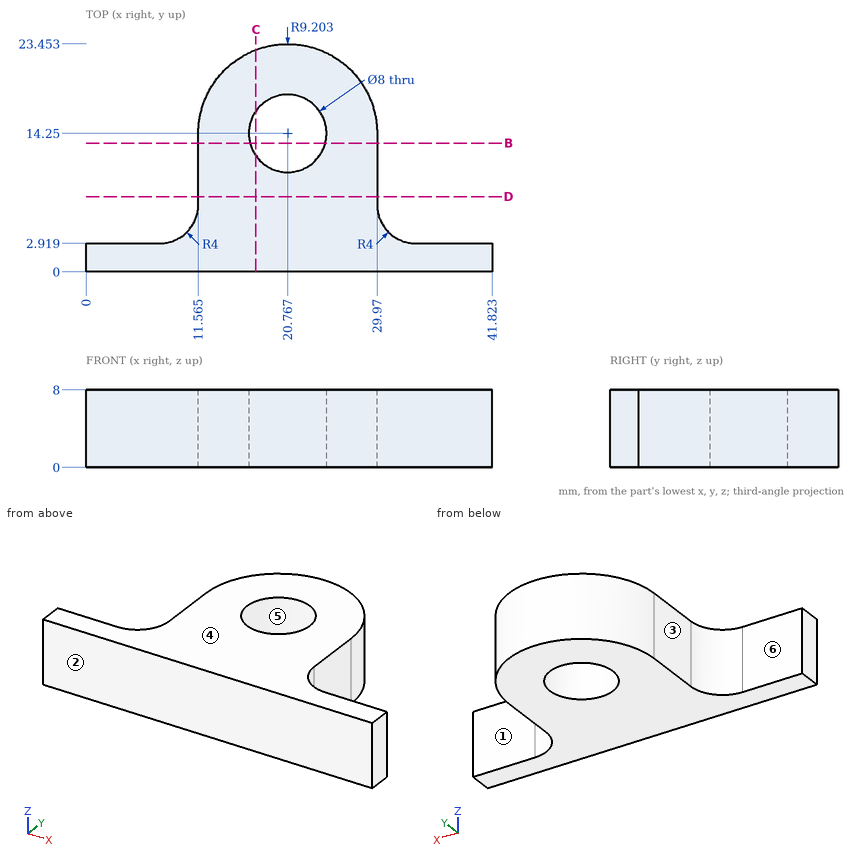
Drawing for the job (mm, zero at the part's lowest x, y, z). A direction names the side the tool comes from. Round coordinates to 2 decimals unless told otherwise and drop trailing zeros. Write each loop counter-clockwise with the first axis right and the second up, starting at its lowest first coordinate (ties: lowest second). Pieces come first, ordered by that corner, then holes. Notation, with made-up numbers: (57.5, 6) - (104.5, 6) arc R21 cw to (104.5, 33) - close; hole circle Ø6 at (83, 68.25). An arc over 180 degrees is marked (long way). Use CSV: the item, a comma, the result in double quotes.
(1) Band-saw the part on D-D (y = 7.75). Write the cut outline in (x, z) (1 decimal).
Response:
outline,"(11.6, 0) - (30, 0) - (30, 8) - (11.6, 8) - close"
(2) Wall check: line 1 (X direction, y = 8.25, z = 5.25) (1 decimal); line 2 (Y direction, x = 21.5, z = 2.5); line 3 (Y direction, x = 18, z = 4.5) (1 decimal). Give the ranges that are in metal, low to high.
Response:
line 1,"11.6 to 30"
line 2,"0 to 10.32, 18.18 to 23.42"
line 3,"0 to 11.4, 17.1 to 23"
(3) Pin check, flat tips, straight feed: P1, Ø2, axis at x = 9, z = 2, coming from the +Y side (1 decimal); P2, Ø1, axis at y = 13.5, z = 5, coming from the +X side; P3, Ø2.5, axis at x = 4.5, z = 2, coming from the +Y side. Stop position of each tip, or through.
Response:
P1,"y = 3.7"
P2,"x = 29.97"
P3,"y = 2.92"
(4) Band-saw the part on C-C (x = 17.5). Write the cut outline in (y, z), plus the area to 3 significant figures.
Response:
outline,"(0, 0) - (11.94, 0) - (11.94, 8) - (0, 8) - close; (16.56, 0) - (22.85, 0) - (22.85, 8) - (16.56, 8) - close"
area,"146 mm²"
(5) 3-axis set-ups, long thin cutter, end or side, ignore diameter. For the marked faces 1, 2 and 3: which of +Z, -Z, +X, -X, +Y, -Y reach the whole face in a straight line?
Response:
face 1,"+Z, -Z, +X, +Y"
face 2,"+Z, -Z, +X, -X, -Y"
face 3,"+Z, -Z, -X, +Y"
(6) Mould opens along Y. For the marked faces 4, 5 and 6 say: pulls with the +Y half, pulls with the -Y half, needs draft (parallel to the pull), parting line crosses it, or undercut.
Response:
face 4,"needs draft"
face 5,"undercut"
face 6,"pulls with the +Y half"
(7) Band-saw the part on B-B (y = 13.25). Write the cut outline in (x, z) (1 decimal).
Response:
outline,"(11.6, 0) - (16.9, 0) - (16.9, 8) - (11.6, 8) - close; (24.6, 0) - (30, 0) - (30, 8) - (24.6, 8) - close"
